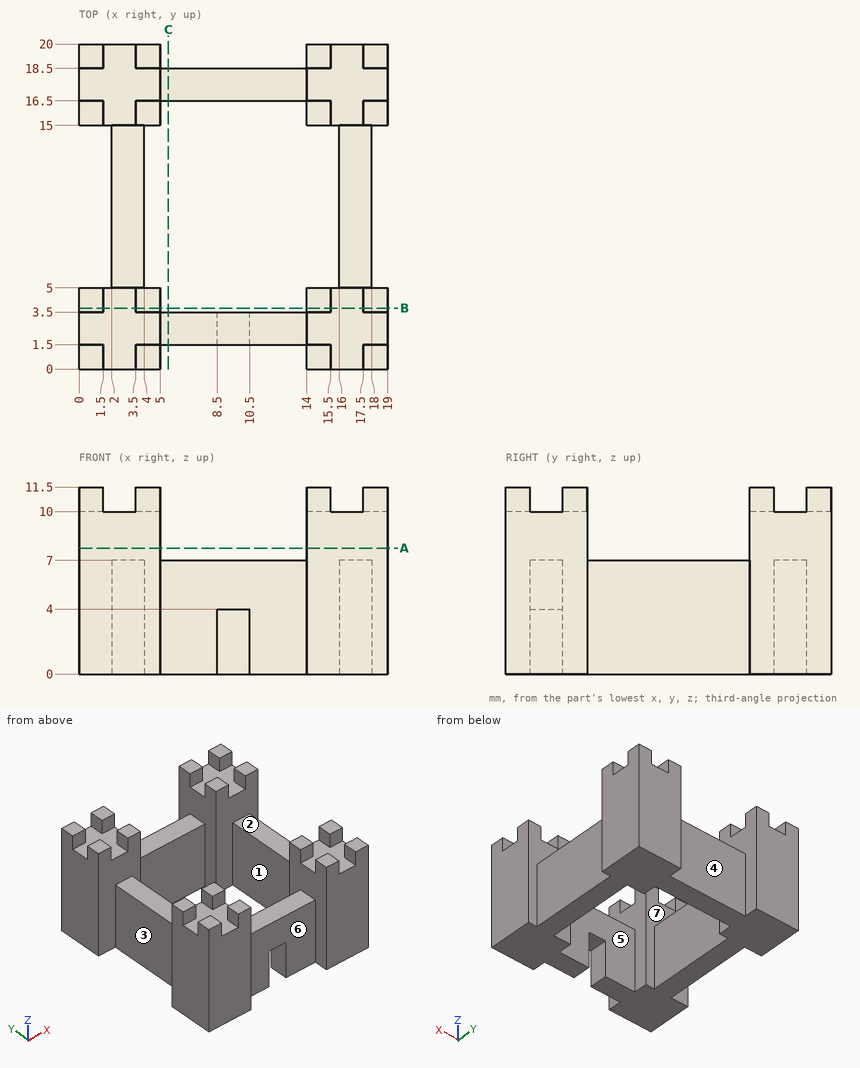
Input: dimensioned drawing with shaded views. Units: mm. Origin: part minimum x, y, z. A direction names the side the tool comes from. Round coordinates to 2 decimals unless told otherwise and drop trailing zeros. Order: outer loops, then holes, each group sorted by start corner. A loop starts at its lowest first (then second) coordinate and runs counter-clockwise, first axis right, second up.
Q1. Mould query, pull axis Y, two halves, no side actions, for the marked faces 4, 5, 6 and 7. Classes: released by +Y, released by -Y, zero draft, split by the parting line, or undercut.
Result sheet:
face 4: released by +Y
face 5: undercut
face 6: released by -Y
face 7: undercut
Q2. Access query for the marked faces 1, 2 and 3. Directions: +Z, -Z, +X, -X, +Y, -Y. A direction counts if a zero-diameter tool reaches every point of the face in a straight line with its end or side. Return the directions, or none.
Result sheet:
face 1: +Z, -Z
face 2: +Z, +X, -X
face 3: +Z, -Z, -X
Q3. Section B-B, the plane y = 3.75. Output: boundary loops of the cut face in (x, z).
Result sheet:
outline: (0, 0) - (5, 0) - (5, 11.5) - (3.5, 11.5) - (3.5, 10) - (1.5, 10) - (1.5, 11.5) - (0, 11.5) - close; (14, 0) - (19, 0) - (19, 11.5) - (17.5, 11.5) - (17.5, 10) - (15.5, 10) - (15.5, 11.5) - (14, 11.5) - close
Q4. Pin query (flat end, axial travel): pin 1 (3 mm diameter, centred on x = 7, z = 2.5, fed in from -Y); pin 2 (1 mm diameter, centred on y = 7.5, z = 4.5, fed in from -X). Return the tip coordinate at first contact, or that it passes through.
Result sheet:
pin 1: stops at y = 1.5
pin 2: stops at x = 2
Q5. Section A-A, the plane z = 7.75. Output: boundary loops of the cut face in (x, y).
Result sheet:
outline: (0, 0) - (5, 0) - (5, 5) - (0, 5) - close; (0, 15) - (5, 15) - (5, 20) - (0, 20) - close; (14, 0) - (19, 0) - (19, 5) - (14, 5) - close; (14, 15) - (19, 15) - (19, 20) - (14, 20) - close
Q6. Section C-C, the plane x = 5.5. Output: boundary loops of the cut face in (y, z), and give its area (3 significant figures).
Result sheet:
outline: (1.5, 0) - (3.5, 0) - (3.5, 7) - (1.5, 7) - close; (16.5, 0) - (18.5, 0) - (18.5, 7) - (16.5, 7) - close
area: 28.0 mm2
Q7. Material intervals for probe 1 along Y at (x, z) = (7.5, 6.5); probe 2 along Y at (x, z) = (1.5, 6.5); probe 3 along Y at (x, z) = (4.5, 11.25), sorted ascending.
Result sheet:
probe 1: y = 1.5 to 3.5, 16.5 to 18.5
probe 2: y = 0 to 5, 15 to 20
probe 3: y = 0 to 1.5, 3.5 to 5, 15 to 16.5, 18.5 to 20
